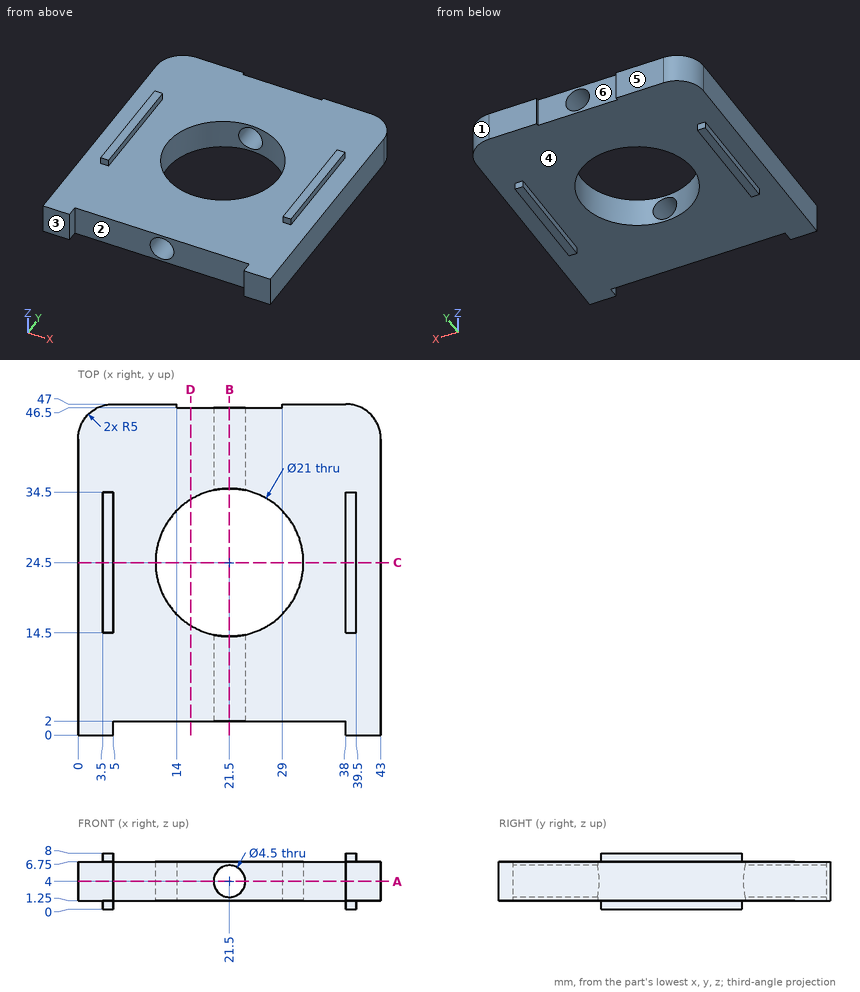
The drawing under review shows one solid part. Ordinate dimensions are in mm from its lowest x, y, z. A direction names the side the tool comes from. Coordinates: 2 decimals unless noted, no trailing zeros. Loops run counter-clockwise (first coordinate to the right, second up) from the corner with the lowest first, then second, coordinate; pieces in that order, holes last.
Item 1: Add section B-B (x = 21.5). Write out the cut boundary in (y, z), and give its area (3 significant figures).
Completed:
outline: (2, 1.25) - (14, 1.25) - (14, 1.75) - (2, 1.75) - close; (2, 6.25) - (14, 6.25) - (14, 6.75) - (2, 6.75) - close; (35, 1.25) - (46.5, 1.25) - (46.5, 1.75) - (35, 1.75) - close; (35, 6.25) - (46.5, 6.25) - (46.5, 6.75) - (35, 6.75) - close
area: 23.5 mm2
Item 2: Add section A-A (z = 4). Write out the cut boundary in (x, y).
Completed:
outline: (0, 0) - (5, 0) - (5, 2) - (19.25, 2) - (19.25, 14.24) arc R10.5 cw to (19.25, 34.76) - (19.25, 46.5) - (14, 46.5) - (14, 47) - (5, 47) arc R5 ccw to (0, 42) - close; (23.75, 2) - (38, 2) - (38, 0) - (43, 0) - (43, 42) arc R5 ccw to (38, 47) - (29, 47) - (29, 46.5) - (23.75, 46.5) - (23.75, 34.76) arc R10.5 cw to (23.75, 14.24) - close
Item 3: Clearance check with flat-ended pins moving along their axes: pin 1 (0.6 mm diameter, centred on x = 4.5, z = 7, fed in from +Y); pin 2 (4.5 mm diameter, centred on x = 19, z = 3.5, fed in from +Y); pin 3 (0.6 mm diameter, centred on y = 21.5, z = 7.5, fed in from -X); pin 4 (2.5 mm diameter, centred on x = 21.5, z = 4, fed in from -Y). State where each tip first meets the part, or that it passes through.
Completed:
pin 1: stops at y = 46.99
pin 2: stops at y = 46.5
pin 3: stops at x = 3.5
pin 4: passes through
Item 4: For the marked faces 5 and 6, list the 3-axis set-ups (+Z, -Z, +X, -X, +Y, -Y) from which the entire face can be reached by the end or side of a thin tool; tool diameter is ignored.
Completed:
face 5: +Z, -Z, +X, -X, +Y
face 6: +Z, -Z, +Y
Item 5: Wall thickness on L1, parallel to X at y = 25, z = 1; L2, parallel to Z at x = 21.5, y = 9; L3, parallel to Y at x = 8, z = 4.75: over which ranges is each line inside the solid? List them lowest first.
Completed:
L1: x = 3.5 to 5, 38 to 39.5
L2: z = 1.25 to 1.75, 6.25 to 6.75
L3: y = 2 to 47
Item 6: Add section D-D (x = 16). Write out the cut boundary in (y, z).
Completed:
outline: (2, 1.25) - (15.56, 1.25) - (15.56, 6.75) - (2, 6.75) - close; (33.44, 1.25) - (46.5, 1.25) - (46.5, 6.75) - (33.44, 6.75) - close
Item 7: Draft analysis for pull direction X (two halves, no side actions). For the marked faces 1, 2, 3 and 4, state which applies: pulls with the +X half, pulls with the -X half, needs draft (parallel to the pull), parting line crosses it, or undercut.
Completed:
face 1: pulls with the +X half
face 2: undercut
face 3: needs draft
face 4: undercut
Item 8: Add section C-C (y = 24.5). Write out the cut boundary in (x, z), and give its area (4 significant figures).
Completed:
outline: (0, 1.25) - (3.5, 1.25) - (3.5, 0) - (5, 0) - (5, 1.25) - (11, 1.25) - (11, 6.75) - (5, 6.75) - (5, 8) - (3.5, 8) - (3.5, 6.75) - (0, 6.75) - close; (32, 1.25) - (38, 1.25) - (38, 0) - (39.5, 0) - (39.5, 1.25) - (43, 1.25) - (43, 6.75) - (39.5, 6.75) - (39.5, 8) - (38, 8) - (38, 6.75) - (32, 6.75) - close
area: 128.5 mm2
